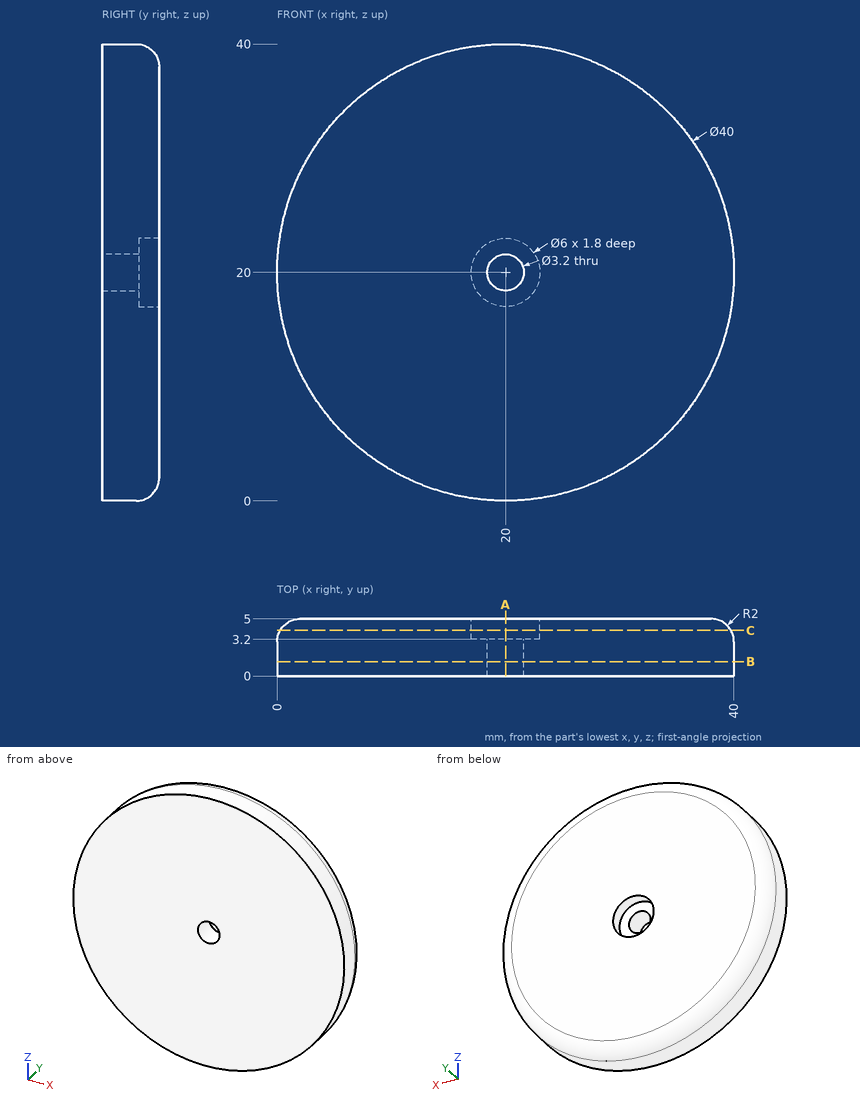
Check sheet for the drawn part. Datum: minimum x, y, z corner. Units: mm. Round coordinates to 2 decimals unless told otherwise and drop trailing zeros. Loops run counter-clockwise (first coordinate to the right, second up) from the corner with the lowest first, then second, coordinate; pieces in that order, holes last. Notation, with made-up numbers: (60.5, 25) - (105.5, 25) arc R19 cw to (105.5, 61) - close; hole circle Ø2 at (43.5, 57). An arc over 180 degrees is marked (long way). Write item = value, one per line. Start each with the question number.
1. Section check B-B on y = 1.25. Enter the section's corners in (x, z).
2. Thickness scan on line 1 (X direction, y = 1.5, z = 20); line 2 (Z direction, x = 21, y = 4.65); line 3 (Z direction, x = 17.5, y = 3.3). Record the ranges inside material, lowest first.
3. Section check A-A on x = 20. Enter the section's corners in (y, z), then the cut area to 3 significant figures.
4. Section check C-C on y = 4. Enter the section's corners in (x, z).
5. Depth check by flat-ended pin: pin 1 (4 mm diameter, centred on x = 6, z = 29.5, fed in from -Y); pin 2 (3 mm diameter, centred on x = 31.5, y = 2.5, fed in from +Z); pin 3 (2 mm diameter, centred on y = 2.5, z = 25.5, fed in from -X); pin 4 (3.5 mm diameter, centred on x = 20, z = 20, fed in from +Y). Enter the tip coordinate at first touch or a pass-through.
Working result:
q1.outline = circle Ø40 at (20, 20); hole circle Ø3.2 at (20, 20)
q2.line_1 = 0 to 18.4, 21.6 to 40
q2.line_2 = 0.9 to 17.17, 22.83 to 39.1
q2.line_3 = 0.18 to 18.34, 21.66 to 39.82
q3.outline = (0, 0) - (3, 0) arc R2 ccw to (5, 2) - (5, 17) - (3.2, 17) - (3.2, 18.4) - (0, 18.4) - close; (0, 21.6) - (3.2, 21.6) - (3.2, 23) - (5, 23) - (5, 38) arc R2 ccw to (3, 40) - (0, 40) - close
q3.area = 177 mm^2
q4.outline = circle Ø39.46 at (20, 20); hole circle Ø6 at (20, 20)
q5.pin_1 = 0
q5.pin_2 = 37.32
q5.pin_3 = 0.51
q5.pin_4 = 3.2
